```python
from build123d import *

# Parameters (mm, degrees)
BOSS_EXTRUDE1_DEPTH          = 1.5
SKETCH2_W                    = 43.5
SKETCH2_H                    = 19.5
BOSS_EXTRUDE2_DEPTH          = 3.5
SKETCH3_W                    = 42
SKETCH3_H                    = 19.5
CUT_EXTRUDE1_DEPTH           = 2
BOSS_EXTRUDE3_DEPTH          = 1.5
F_8_0_8_DIAMETER_HOLE1_D     = 8
F_8_0_8_DIAMETER_HOLE1_DEPTH = 1.5
F_8_0_8_DIAMETER_HOLE2_D     = 8
F_8_0_8_DIAMETER_HOLE2_DEPTH = 1.5
FILLET1_R                    = 0.5
FILLET2_R                    = 2
SKETCH9_W                    = 25
SKETCH9_H                    = 6
CUT_EXTRUDE2_DEPTH           = 1.5
FILLET3_R                    = 0.5
CUT_EXTRUDE3_DEPTH           = 45
FILLET4_R                    = 0.5


with BuildPart() as part:
    # Sketch1 → Boss-Extrude1 (new body)
    with BuildSketch(Plane(origin=(-22.5, 0, 0), x_dir=(0, -1, 0), z_dir=(-1, 0, 0))):
        with BuildLine():
            Line((82.02741971, -6.037413385), (58.5, 13.5))
            Line((58.5, 13.5), (39, 13.5))
            Line((39, 13.5), (-0.697466415, 10.97786594))
            ThreePointArc((-0.697466415, 10.97786594), (-10.994465093, -0.348908769), (0, -11))
            Line((0, -11), (50, -11))
            Line((50, -11), (68.880323706, -23.640544954))
            ThreePointArc((68.880323706, -23.640544954), (83.813260452, -21.082282295), (82.02741971, -6.037413385))
        make_face()
    extrude(amount=-BOSS_EXTRUDE1_DEPTH)

    # Sketch2 → Boss-Extrude2 (add)
    with BuildSketch(Plane.XY.offset(13.5)):
        with Locations((-0.75, -48.75)):
            Rectangle(SKETCH2_W, SKETCH2_H)
    extrude(amount=BOSS_EXTRUDE2_DEPTH)

    # Sketch3 → Cut-Extrude1 (cut)
    with BuildSketch(Plane(origin=(0, 0, 13.5), x_dir=(-1, 0, 0), z_dir=(0, 0, -1))):
        with Locations((0, -48.75)):
            Rectangle(SKETCH3_W, SKETCH3_H)
    extrude(amount=-CUT_EXTRUDE1_DEPTH, mode=Mode.SUBTRACT)

    # Sketch4 → Boss-Extrude3 (add)
    with BuildSketch(Plane(origin=(21, 0, 0), x_dir=(0, 0, -1), z_dir=(1, 0, 0))):
        with BuildLine():
            Line((11, 0), (11, -50))
            Line((11, -50), (23.640544954, -68.880323706))
            ThreePointArc((23.640544954, -68.880323706), (21.082282295, -83.813260452), (6.037413385, -82.02741971))
            Line((6.037413385, -82.02741971), (-13.5, -58.5))
            Line((-13.5, -58.5), (-17, -58.5))
            Line((-17, -58.5), (-17, -39))
            Line((-17, -39), (-13.5, -39))
            Line((-13.5, -39), (-10.97786594, 0.697466415))
            ThreePointArc((-10.97786594, 0.697466415), (0.348908769, 10.994465093), (11, 0))
        make_face()
    extrude(amount=BOSS_EXTRUDE3_DEPTH)

    # Ø8.0 (8) Diameter Hole1
    with Locations(Plane.ZY.offset(-21)):
        with Locations((-14.5, -75), (0, 0)):
            Hole(F_8_0_8_DIAMETER_HOLE1_D / 2, depth=F_8_0_8_DIAMETER_HOLE1_DEPTH)

    # Ø8.0 (8) Diameter Hole2
    with Locations(Plane(origin=(-21, 0, 0), x_dir=(0, 0, -1), z_dir=(1, 0, 0))):
        with Locations((14.5, -75), (0, 0)):
            Hole(F_8_0_8_DIAMETER_HOLE2_D / 2, depth=F_8_0_8_DIAMETER_HOLE2_DEPTH)

    # Fillet1
    fillet1_edges = [part.edges().sort_by_distance(p)[0] for p in [
        (21, -48.75, 15.5),
        (-21, -48.75, 15.5),
    ]]
    fillet(fillet1_edges, radius=FILLET1_R)

    # Fillet2
    fillet2_edges = [part.edges().sort_by_distance(p)[0] for p in [
        (-22.5, -48.75, 17),
        (22.5, -48.75, 17),
    ]]
    fillet(fillet2_edges, radius=FILLET2_R)

    # Sketch9 → Cut-Extrude2 (cut)
    with BuildSketch(Plane.XY.offset(17)):
        with Locations((0, -48.75)):
            Rectangle(SKETCH9_W, SKETCH9_H)
    extrude(amount=-CUT_EXTRUDE2_DEPTH, mode=Mode.SUBTRACT)

    # Fillet3
    fillet3_edges = [part.edges().sort_by_distance(p)[0] for p in [
        (12.5, -51.75, 16.25),
        (-12.5, -51.75, 16.25),
        (-12.5, -45.75, 16.25),
        (12.5, -45.75, 16.25),
    ]]
    fillet(fillet3_edges, radius=FILLET3_R)

    # Sketch11 → Cut-Extrude3 (cut)
    with BuildSketch(Plane.ZY.offset(22.5)):
        Polygon((-0.103461549, -47.005534907), (5.033080081, -46.962059996), (4.939981079, -35.962453976), (-0.150011884, -36.005534907), (-5.240187158, -36.005534907), (-5.240187158, -47.005534907), align=None)
        Polygon((-0.22195331, -19.005534907), (-5.22195331, -19.005534907), (-5.22195331, -30.005534907), (-0.175402975, -30.005534907), (4.87096661, -29.962823198), (4.777867607, -18.963217179), align=None)
    extrude(amount=-CUT_EXTRUDE3_DEPTH, mode=Mode.SUBTRACT)

    # Fillet4
    fillet4_edges = [part.edges().sort_by_distance(p)[0] for p in [
        (-21.75, -36.005534907, -0.150011884),
        (-21.75, -35.962453976, 4.939981079),
        (-21.75, -46.962059996, 5.033080081),
        (-21.75, -47.005534907, -0.103461549),
        (-21.75, -47.005534907, -5.240187158),
        (-21.75, -36.005534907, -5.240187158),
        (21.75, -36.005534907, -0.150011884),
        (21.75, -35.962453976, 4.939981079),
        (21.75, -46.962059996, 5.033080081),
        (21.75, -47.005534907, -0.103461549),
        (21.75, -47.005534907, -5.240187158),
        (21.75, -36.005534907, -5.240187158),
        (-21.75, -19.005534907, -0.22195331),
        (-21.75, -18.963217179, 4.777867607),
        (-21.75, -29.962823198, 4.87096661),
        (-21.75, -30.005534907, -0.175402975),
        (-21.75, -30.005534907, -5.22195331),
        (-21.75, -19.005534907, -5.22195331),
        (21.75, -19.005534907, -0.22195331),
        (21.75, -18.963217179, 4.777867607),
        (21.75, -29.962823198, 4.87096661),
        (21.75, -30.005534907, -0.175402975),
        (21.75, -30.005534907, -5.22195331),
        (21.75, -19.005534907, -5.22195331),
    ]]
    fillet(fillet4_edges, radius=FILLET4_R)


solid = part.part
```
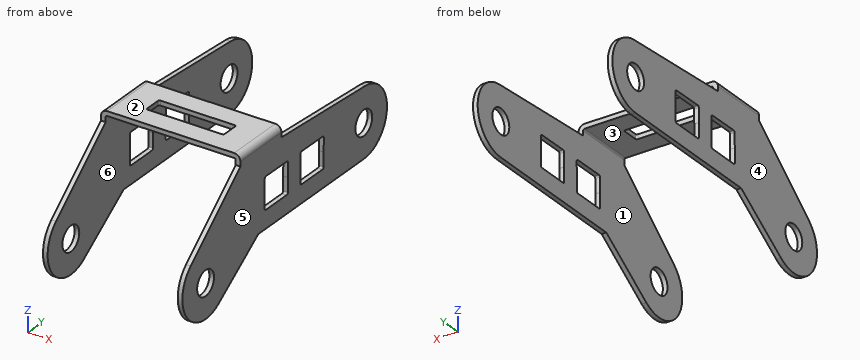
Build history of the part. All positions in model axes, mm. Face numbers are marked on the shaded views. A direction names the side the tool comes from. Round coordinates to 2 decimals unless told otherwise and drop trailing zeros. Order: outer loops, then holes, each group sorted by start corner. A loop starts at its lowest first (then second) coordinate and runs counter-clockwise, first axis right, second up. Notation, with made-up numbers: (32, -1.5) -> (39, -1.5) arc R23 ccw to (39, 11.5) -> close; hole circle Ø5 at (80.5, -12.75). An arc over 180 degrees is marked (long way). Answer in a Markdown table with one row per item.
1) Pin check, flat tips, straight feed: P1, Ø1.6, axis at x = -21.5, z = -1.5, coming from the +Y side; P2, Ø1.6, axis at x = -21.5, z = -2.5, coming from the +Y side; P3, Ø0.8, axis at x = 21.5, y = -41, coming from the +Z side. Stop position of each tip, or through.
Values:
| item | result |
|---|---|
| P1 | y = 10.98 |
| P2 | y = 10.87 |
| P3 | z = 16.91 |
2) Mould opens along X. For the marked faces 3, 4, 5 and 6 say: released by +X, released by -X, zero draft, split by the parting line, or undercut.
Values:
| item | result |
|---|---|
| face 3 | undercut |
| face 4 | released by -X |
| face 5 | released by +X |
| face 6 | undercut |
3) Band-saw the part on B-B on z = -21. Give the cut face in (x, y), and give its area (3 significant figures).
Values:
| item | result |
|---|---|
| outline | (-22.5, -83.87) -> (-21, -83.87) -> (-21, -64.94) -> (-22.5, -64.94) -> close; (21, -83.87) -> (22.5, -83.87) -> (22.5, -64.94) -> (21, -64.94) -> close |
| area | 56.8 mm2 |
4) Band-saw the part on C-C on y = -77.5. Give the cut face in (x, z), and give its area (3 significant figures).
Values:
| item | result |
|---|---|
| outline | (-22.5, -25.21) -> (-21, -25.21) -> (-21, -17.62) -> (-22.5, -17.62) -> close; (-22.5, -11.38) -> (-21, -11.38) -> (-21, -2.28) -> (-22.5, -2.28) -> close; (21, -25.21) -> (22.5, -25.21) -> (22.5, -17.62) -> (21, -17.62) -> close; (21, -11.38) -> (22.5, -11.38) -> (22.5, -2.28) -> (21, -2.28) -> close |
| area | 50.1 mm2 |
5) Which spindle directions (+Z, -Z, +X, -X, +Y, -Y) get a long thin tool onto all of the face, cutting with end or side? Do the marked faces 1 and 2. Say none if no direction does.
Values:
| item | result |
|---|---|
| face 1 | -Z, +Y, -Y |
| face 2 | +Z, +X, -X, +Y, -Y |
6) Band-saw the part on A-A on x = 3. Give the cut face in (y, z).
Values:
| item | result |
|---|---|
| outline | (-58.5, 15.5) -> (-51.75, 15.5) -> (-51.75, 17) -> (-58.5, 17) -> close; (-45.75, 15.5) -> (-39, 15.5) -> (-39, 17) -> (-45.75, 17) -> close |
7) Wall check: L1, parallel to X at y = -60.5, z = -10; L2, parallel to Y at x = -21.4, z = 0; L3, parallel to Y at x = -22, z = -14. Give the ranges that are in metal, low to high.
Values:
| item | result |
|---|---|
| L1 | -22.5 to -21, 21 to 22.5 |
| L2 | -74.76 to -47, -36 to -30, -19 to -4, 4 to 11 |
| L3 | -85.99 to -78.97, -71.03 to -54.48 |
8) Band-saw the part on D-D on z = -14.5. Give the cut face in (x, y), and give its area (3 significant figures).
Values:
| item | result |
|---|---|
| outline | (-22.5, -86) -> (-21, -86) -> (-21, -79) -> (-22.5, -79) -> close; (-22.5, -71) -> (-21, -71) -> (-21, -55.23) -> (-22.5, -55.23) -> close; (21, -86) -> (22.5, -86) -> (22.5, -79) -> (21, -79) -> close; (21, -71) -> (22.5, -71) -> (22.5, -55.23) -> (21, -55.23) -> close |
| area | 68.3 mm2 |
